Answer from the drawing. Dimensions are ordinates in mm from the lowest x, y and z of the part. Give positions to 0.01 mm unless a question says otherwise; leave off trailing zeros. Loops run counter-clockwise (first coordinate to the right, second up) from the corner with the lowest first, then second, coordinate; pieces in that order, holes last. Notation, with made-up numbers: M 10,84.5 L 31,84.5 A34 cw 31,121.5 Z; hole C -10,22 d3. An arc over 180 degrees is marked long. Use a Markdown table: item, result.
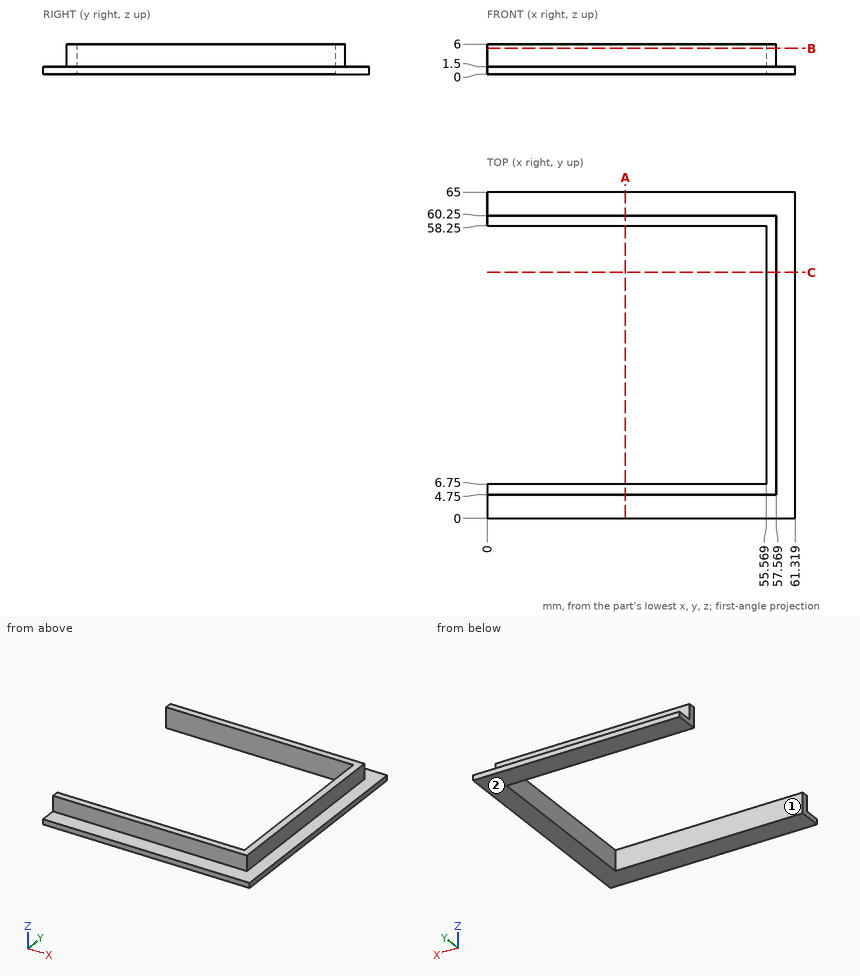
(1) A cutting plane is placed at A-A (x = 27.5). Write down the section's boundary in (y, z).
Entries:
| item | result |
|---|---|
| outline | M 0,0 L 6.75,0 L 6.75,6 L 4.75,6 L 4.75,1.5 L 0,1.5 Z; M 58.25,0 L 65,0 L 65,1.5 L 60.25,1.5 L 60.25,6 L 58.25,6 Z |
(2) A cutting plane is placed at B-B (z = 5.15). Write down the section's boundary in (x, y).
Entries:
| item | result |
|---|---|
| outline | M 0,4.75 L 57.57,4.75 L 57.57,60.25 L 0,60.25 L 0,58.25 L 55.57,58.25 L 55.57,6.75 L 0,6.75 Z |
(3) A cutting plane is placed at C-C (y = 49). Write down the section's boundary in (x, z).
Entries:
| item | result |
|---|---|
| outline | M 55.57,0 L 61.32,0 L 61.32,1.5 L 57.57,1.5 L 57.57,6 L 55.57,6 Z |
(4) The mould has two halves that part along Y. Classify the marked faces 1 and 2: released by +Y, released by -Y, zero draft, split by the parting line, or undercut.
Entries:
| item | result |
|---|---|
| face 1 | undercut |
| face 2 | zero draft |
(5) Consider probe 1 along Y at (x, z) = (19, 4.5); probe 2 along X at (y, z) = (28.5, 1.2); probe 3 along X at (y, z) = (42, 5.5). Determine where each line is inside the solid, lowest interval first. Write a range as [from, to].
Entries:
| item | result |
|---|---|
| probe 1 | y = [4.75, 6.75], [58.25, 60.25] |
| probe 2 | x = [55.57, 61.32] |
| probe 3 | x = [55.57, 57.57] |
(6) Given P1, Ø2, axis at y = 29, z = 3, coming from the +X side; P2, Ø1.8, axis at y = 35, z = 4, coming from the -X side; P3, Ø2, axis at x = 35.5, z = 3.5, coming from the +Y side; P4, Ø6, axis at x = 37, y = 55, coming from the +Z side, each flat-ended and moving along its own axis, determine where each tip first touches the part or whether it passes through.
Entries:
| item | result |
|---|---|
| P1 | stops at x = 57.57 |
| P2 | stops at x = 55.57 |
| P3 | stops at y = 60.25 |
| P4 | passes through |
